Verification items for the finished model (mm, model axes). A direction names the side the tool comes from. Coordinates: 2 decimals unless noted, no trailing zeros. Order: outer loops, then holes, each group sorted by start corner. A loop starts at its lowest first (then second) coordinate and runs counter-clockwise, first axis right, second up. Notation, with made-up numbers: (5, -23) -> (46, -23) arc R18 cw to (46, 3) -> close; hole circle Ø8 at (74, 58.5). An arc over 180 degrees is marked (long way). Use CSV: the item, a comma, the result in double quotes. Start each with the question number.
1) Go/stop test with flat-tipped pins: pin 1 (12.5 mm diameter, centred on x = 35, y = -32.5, fed in from +Z); pin 2 (3 mm diameter, centred on x = -5.5, z = -9, fed in from -Y); pin 3 (2 mm diameter, centred on y = -16.5, z = 19.5, fed in from -X). Record where each tip stops, or that it passes through.
2) Tool access check on faces 5 (the flat face through (-1, -38, 47.171)), 6 (the flat face through (-1, -38, 96.777)), 7 (the flat face through (95.634, -38, -1)). Record the directions out of +Z, -Z, +X, -X, +Y, -Y that give a thin tool (end or side, any length) a straight path to the whole face; none if there is none.
3) Sectioned sample at B-B on z = -19.5. Record the boundary of the cut face in (x, y).
4) Sectioned sample at C-C on x = 18. Record the boundary of the cut face in (y, z), then the cut area to 3 significant figures.
5) Scan lines: line 1 along X through (y, z) = (-29, 32); line 2 along Z through (x, y) = (-16.5, -35.5); line 3 along Z through (x, y) = (83.5, -46). Record each from-to range of solid material in increasing order.
6) Sectioned sample at A-A on y = -31.5. Record the boundary of the cut face in (x, z).
7) Release check for a two-part mould opening along X. For faces 1 (the flat face through (-95.353, 0, 0)), 2 (the flat face through (1, 25.4, 2)), 3 (the flat face through (95.634, 0, 0)), 4 (the flat face through (44.717, -38, -1)) record: released by +X, released by -X, zero draft, split by the parting line, or undercut.
from build123d import *

# Parameters (mm, degrees)
F0_W     = 190.987497
F0_H     = 195.329547
F1_DEPTH = 25.4
F2_W     = 190.987497
F2_H     = 195.329547
F2_W_2   = 92.081398
F2_H_2   = 90.176002
F3_DEPTH = 25.4
F4_W     = 191.268652
F4_H     = 193.553298
F4_W_2   = 89.433506
F4_H_2   = 94.341778
F5_DEPTH = 25.4
F6_W     = 92.081398
F6_H     = 90.176002
F7_DEPTH = 25.4


with BuildPart() as f1:
    # F0 (on Front) → F1 (new body)
    with BuildSketch(Plane.XZ):
        with Locations((0.140578, 0.888125)):
            Rectangle(F0_W, F0_H)
    extrude(amount=F1_DEPTH)

    # F2 (on face) → F3 (join)
    with BuildSketch(Plane(origin=(0, 0, 0), x_dir=(-1, 0, 0), z_dir=(0, 1, 0))):
        with Locations((-0.140578, 0.888125)):
            Rectangle(F2_W, F2_H)
        Rectangle(F2_W_2, F2_H_2, mode=Mode.SUBTRACT)
    extrude(amount=F3_DEPTH)

    # F4 (on face) → F5 (join)
    with BuildSketch(Plane.XZ.offset(25.4)):
        Rectangle(F4_W, F4_H)
        Rectangle(F4_W_2, F4_H_2, mode=Mode.SUBTRACT)
    extrude(amount=F5_DEPTH)

    # F6 (on face) → F7 (join)
    with BuildSketch(Plane(origin=(0, 0, 0), x_dir=(-1, 0, 0), z_dir=(0, 1, 0))):
        Rectangle(F6_W, F6_H)
    extrude(amount=F7_DEPTH)


solid = f1.part
Answers follow:
1,pin 1,"stops at z = 96.78"
1,pin 2,"stops at y = -25.4"
1,pin 3,"stops at x = -95.35"
2,face 5,"-Y"
2,face 6,"+Z, +X, -X, -Y"
2,face 7,"+Z, -Z, +X, +Y, -Y"
3,outline,"(-95.63, -50.8) -> (-44.72, -50.8) -> (-44.72, -25.4) -> (44.72, -25.4) -> (44.72, -50.8) -> (95.63, -50.8) -> (95.63, 25.4) -> (-95.35, 25.4) -> (-95.35, -25.4) -> (-95.63, -25.4) -> close"
4,outline,"(-50.8, -96.78) -> (25.4, -96.78) -> (25.4, 98.55) -> (-25.4, 98.55) -> (-25.4, 96.78) -> (-50.8, 96.78) -> (-50.8, 47.17) -> (-25.4, 47.17) -> (-25.4, -47.17) -> (-50.8, -47.17) -> close"
4,area,"12,400 mm²"
5,line 1,"x = -95.63 to -44.72, 44.72 to 95.63"
5,line 2,"z = -96.78 to -47.17, 47.17 to 96.78"
5,line 3,"z = -96.78 to 96.78"
6,outline,"(-95.63, -96.78) -> (95.63, -96.78) -> (95.63, 96.78) -> (-95.63, 96.78) -> close; hole (-44.72, -47.17) -> (44.72, -47.17) -> (44.72, 47.17) -> (-44.72, 47.17) -> close"
7,face 1,"released by -X"
7,face 2,"zero draft"
7,face 3,"released by +X"
7,face 4,"undercut"
